```python
from build123d import *

# Parameters (mm, degrees)
SKETCH1_W               = 127
SKETCH1_H               = 76.2
BOSS_EXTRUDE1_DEPTH     = 6.35
SKETCH3_R               = 5.125
SKETCH3_W               = 50.8
SKETCH3_H               = 30.48
SKETCH3_W_2             = 5
SKETCH3_H_2             = 1
CUT_EXTRUDE1_DEPTH      = 75.324844433
FILLET1_R               = 6.096
SKETCH4_R               = 0.75
CUT_EXTRUDE2_DEPTH      = 19.05
F_1_4_20_TAPPED_HOLE1_D = 5.1054


with BuildPart() as part:
    # Sketch1 → Boss-Extrude1 (new body)
    with BuildSketch(Plane(origin=(0, 0, 0), x_dir=(1, 0, 0), z_dir=(0, 1, 0))):
        Rectangle(SKETCH1_W, SKETCH1_H)
    extrude(amount=BOSS_EXTRUDE1_DEPTH)

    # Sketch3 → Cut-Extrude1 (cut, through all)
    with BuildSketch(Plane(origin=(0, 6.35, 0), x_dir=(1, 0, 0), z_dir=(0, 1, 0))):
        with Locations(Location((0, 0, 0), (0, 0, 270))):
            Circle(SKETCH3_R)
        with Locations((0, -22.86)):
            Rectangle(SKETCH3_W, SKETCH3_H)
        with Locations((10.2, -4.625)):
            Rectangle(SKETCH3_W_2, SKETCH3_H_2)
        with Locations((-10.2, 4.625)):
            Rectangle(SKETCH3_W_2, SKETCH3_H_2)
    extrude(amount=-CUT_EXTRUDE1_DEPTH, mode=Mode.SUBTRACT)

    # Fillet1
    fillet1_edges = [part.edges().sort_by_distance(p)[0] for p in [
        (-25.4, 3.175, 7.62),
        (25.4, 3.175, 7.62),
    ]]
    fillet(fillet1_edges, radius=FILLET1_R)

    # Sketch4 → Cut-Extrude2 (cut)
    with BuildSketch(Plane.XY.offset(7.62)):
        with Locations((-10.2, 3.175)):
            Circle(SKETCH4_R)
        with Locations((10.2, 3.175)):
            Circle(SKETCH4_R)
    extrude(amount=-CUT_EXTRUDE2_DEPTH, mode=Mode.SUBTRACT)

    # 1/4-20 Tapped Hole1 (through all)
    with Locations(Plane(origin=(0, 6.35, 0), x_dir=(1, 0, 0), z_dir=(0, 1, 0))):
        with Locations((-50.8, 25.4), (50.8, 25.4), (50.8, -25.4), (-50.8, -25.4)):
            Hole(F_1_4_20_TAPPED_HOLE1_D / 2)


solid = part.part
```
CAD build for the part. Positions are in the model's coordinates, mm. A direction names the side the tool comes from. Coordinates: 2 decimals unless noted, no trailing zeros. Loops run counter-clockwise (first coordinate to the right, second up) from the corner with the lowest first, then second, coordinate; pieces in that order, holes last. Notation, with made-up numbers: (77, 32.5) - (108, 32.5) arc R30 cw to (108, 58.5) - close; hole circle Ø9 at (76.5, 87.5). An arc over 180 degrees is marked (long way). Use CSV: the item, a comma, the result in double quotes. Start each with the question number.
Q1. Two-plate mould, pull along X, no slides. Class faces 1 (the flat face through (-63.5, 3, 1)), 2 (the flat face through (-1, 3, -38.1)), 3 (the cylindrical face through (-5.003, 3.219, -1.111)), 4 (the flat face through (63.5, 3, 1)): +X half, -X half, draft (parallel to the pull), parting line (faces both ways), or undercut.
Q2. Drop a flat-ended pin along its axis: P1, Ø0.8, axis at x = -10.5, y = 3.5, coming from the +Z side. Give the stop position or say it passes through.
Q3. Cut at C-C, the plane x = 50.8. List the corners of the cut face in (y, z), then the cut area to 3 significant figures.
Q4. Probe probe 1 along X at (y, z) = (3, -11); probe 2 along Z at (x, y) = (51, 4.25); probe 3 along Z at (x, y) = (50.8, 2.75). List the from-to ranges inside material, lowest first. Write a range as from..to.
Q5. Cut at A-A, the plane x = 0. List the corners of the cut face in (y, z) (3 decimals), then the cut area to 3 significant figures.
Q6. Cut at B-B, the plane z = 18.5. List the corners of the cut face in (x, y), then the cut area to 3 significant figures.
Q7. Cut at D-D, the plane z = -25.4. List the corners of the cut face in (x, y).
Q8. 3-axis set-ups, long thin cutter, end or side, ignore diameter. For faces 5 (the flat face through (-25.4, 3, 26)), 6 (the flat face through (44, 3, 38.1)), 7 (the flat face through (-11, 4, -5.125)): which of +Z, -Z, +X, -X, +Y, -Y reach the whole face in a straight line?
Here are the results:
1,face 1,"-X half"
1,face 2,"draft"
1,face 3,"undercut"
1,face 4,"+X half"
2,P1,"z = 7.62"
3,outline,"(0, -38.1) - (6.35, -38.1) - (6.35, -27.95) - (0, -27.95) - close; (0, -22.85) - (6.35, -22.85) - (6.35, 22.85) - (0, 22.85) - close; (0, 27.95) - (6.35, 27.95) - (6.35, 38.1) - (0, 38.1) - close"
3,area,"419 mm2"
4,probe 1,"-63.5..-10.93, -9.47..9.47, 10.93..63.5"
4,probe 2,"-38.1..-27.94, -22.86..22.86, 27.94..38.1"
4,probe 3,"-38.1..-27.95, -22.85..22.85, 27.95..38.1"
5,outline,"(0, -38.1) - (6.35, -38.1) - (6.35, -5.125) - (0, -5.125) - close; (0, 5.125) - (6.35, 5.125) - (6.35, 7.62) - (0, 7.62) - close"
5,area,"225 mm2"
6,outline,"(-63.5, 0) - (-25.4, 0) - (-25.4, 6.35) - (-63.5, 6.35) - close; (25.4, 0) - (63.5, 0) - (63.5, 6.35) - (25.4, 6.35) - close"
6,area,"484 mm2"
7,outline,"(-63.5, 0) - (-53.35, 0) - (-53.35, 6.35) - (-63.5, 6.35) - close; (-48.25, 0) - (48.25, 0) - (48.25, 6.35) - (-48.25, 6.35) - close; (53.35, 0) - (63.5, 0) - (63.5, 6.35) - (53.35, 6.35) - close"
8,face 5,"+Z, +Y, -Y"
8,face 6,"+Z, +X, -X, +Y, -Y"
8,face 7,"+Y, -Y"
